Design review of the part built by this model. Coordinates are the model's own, in mm. Face numbers are marked on the shaded views. A direction names the side the tool comes from. Coordinates: 2 decimals unless noted, no trailing zeros. Loops run counter-clockwise (first coordinate to the right, second up) from the corner with the lowest first, then second, coordinate; pieces in that order, holes last. Notation, with made-up numbers: (-5, -15) -> (29, -15) arc R25 cw to (29, 7) -> close; hole circle Ø11 at (39.5, 38). An arc over 180 degrees is marked (long way). Answer as a JSON object with one key per item and string values.
```python
from build123d import *

# Parameters (mm, degrees)
BOSS_EXTRU_1_DEPTH      = 20
ESQUISSE2_R             = 1.25
ENL_V_MAT_EXTRU_1_DEPTH = 8
CONG_1_R                = 10
ESQUISSE3_R             = 2.5
ENL_V_MAT_EXTRU_2_DEPTH = 30


with BuildPart() as part:
    # Esquisse1 → Boss.-Extru.1 (new body)
    with BuildSketch(Plane.XY):
        with BuildLine():
            Line((-15, -0.5), (-15, -10))
            Line((-15, -10), (-12, -10))
            Line((-12, -10), (-12, -30))
            Line((-12, -30), (-9, -30))
            Line((-9, -30), (-9, -10))
            Line((-9, -10), (-6, -10))
            Line((-6, -10), (-6, -30))
            Line((-6, -30), (-3, -30))
            Line((-3, -30), (-3, -10))
            Line((-3, -10), (0, -10))
            Line((0, -10), (0, -30))
            Line((0, -30), (3, -30))
            Line((3, -30), (3, -10))
            Line((3, -10), (6, -10))
            Line((6, -10), (6, -30))
            Line((6, -30), (9, -30))
            Line((9, -30), (9, -10))
            Line((9, -10), (12, -10))
            Line((12, -10), (12, -30))
            Line((12, -30), (15, -30))
            Line((15, -30), (15, -0.5))
            Line((15, -0.5), (5.979130372, -0.5))
            ThreePointArc((5.979130372, -0.5), (0, -6), (-5.979130372, -0.5))
            Line((-5.979130372, -0.5), (-15, -0.5))
        make_face()
    extrude(amount=BOSS_EXTRU_1_DEPTH)

    # Esquisse2 → Enlèv. mat.-Extru.1 (cut)
    with BuildSketch(Plane(origin=(0, -0.5, 0), x_dir=(1, 0, 0), z_dir=(0, 1, 0))):
        with Locations(Location((-10, -5, 0), (0, 0, 180))):
            Circle(ESQUISSE2_R)
        with Locations(Location((-10, -15, 0), (0, 0, 180))):
            Circle(ESQUISSE2_R)
        with Locations(Location((10, -5, 0), (0, 0, 180))):
            Circle(ESQUISSE2_R)
        with Locations(Location((10, -15, 0), (0, 0, 180))):
            Circle(ESQUISSE2_R)
    extrude(amount=-ENL_V_MAT_EXTRU_1_DEPTH, mode=Mode.SUBTRACT)

    # Congé1
    cong_1_edges = [part.edges().sort_by_distance(p)[0] for p in [
        (-10.5, -30, 0),
        (-4.5, -30, 0),
        (1.5, -30, 0),
        (7.5, -30, 0),
        (13.5, -30, 0),
        (13.5, -30, 20),
        (7.5, -30, 20),
        (1.5, -30, 20),
        (-4.5, -30, 20),
        (-10.5, -30, 20),
    ]]
    fillet(cong_1_edges, radius=CONG_1_R - 0.0001)  # a hair under: the kernel refuses the full size

    # Esquisse3 → Enlèv. mat.-Extru.2 (cut)
    with BuildSketch(Plane(origin=(15, 0, 0), x_dir=(0, 0, -1), z_dir=(1, 0, 0))):
        with Locations(Location((-10, -20, 0), (0, 0, 90))):
            Circle(ESQUISSE3_R)
    extrude(amount=-ENL_V_MAT_EXTRU_2_DEPTH, mode=Mode.SUBTRACT)


solid = part.part
```
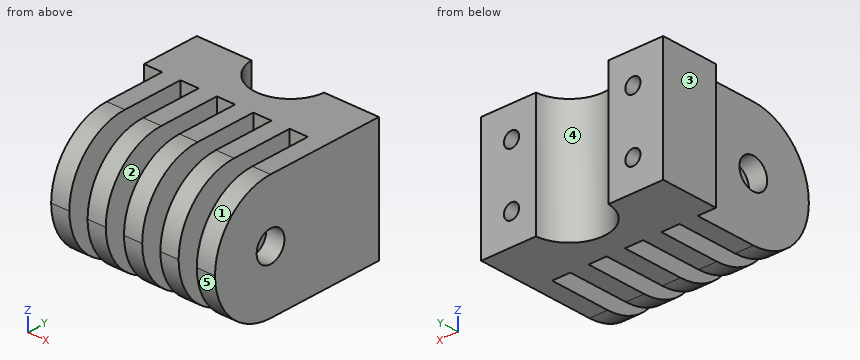
1) For the marked faces 1 and 2, list the 3-axis set-ups (+Z, -Z, +X, -X, +Y, -Y) from which the entire face can be reached by the end or side of a thin tool; tool diameter is ignored.
Completed:
{"face 1": "+Z, +X, -X, -Y", "face 2": "+Z, -Z, -Y"}
2) Add section D-D, the plane z = 18.25. Give the boundary of the cut face in (x, y), and give its area (3 significant figures).
Completed:
{"outline": "(-15, -10) -> (-12, -10) -> (-12, -25.65) -> (-9, -25.65) -> (-9, -10) -> (-6, -10) -> (-6, -25.65) -> (-3, -25.65) -> (-3, -10) -> (0, -10) -> (0, -25.65) -> (3, -25.65) -> (3, -10) -> (6, -10) -> (6, -25.65) -> (9, -25.65) -> (9, -10) -> (12, -10) -> (12, -25.65) -> (15, -25.65) -> (15, -0.5) -> (5.98, -0.5) arc R6 cw to (-5.98, -0.5) -> (-15, -0.5) -> close", "area": "469 mm²"}
3) Add section A-A, the plane y = -15.5. Give the boundary of the cut face in (x, z).
Completed:
{"outline": "(-12, 0) -> (-9, 0) -> (-9, 20) -> (-12, 20) -> close; (-6, 0) -> (-3, 0) -> (-3, 20) -> (-6, 20) -> close; (0, 0) -> (3, 0) -> (3, 20) -> (0, 20) -> close; (6, 0) -> (9, 0) -> (9, 20) -> (6, 20) -> close; (12, 0) -> (15, 0) -> (15, 20) -> (12, 20) -> close"}
4) Clearance check with flat-ended pins moving along their axes: pin 1 Ø1.5 at (y, z) = (-12.5, 10.5) entering from -X; pin 2 Ø4.5 at (y, z) = (-20, 10) entering from +X (3 decimals); pin 3 Ø3 at (x, z) = (-9.5, 15) entering from +Y; pin 4 Ø2 at (x, z) = (10, 15) entering from +Y. State where each tip first meets the part, or that it passes through.
Completed:
{"pin 1": "x = -12", "pin 2": "through", "pin 3": "y = -0.5", "pin 4": "y = -8.5"}
5) Add section C-C, the plane x = 10. Give the boundary of the cut face in (y, z), and give its area (3 significant figures).
Completed:
{"outline": "(-10, 0) -> (-0.5, 0) -> (-0.5, 3.75) -> (-8.5, 3.75) -> (-8.5, 6.25) -> (-0.5, 6.25) -> (-0.5, 13.75) -> (-8.5, 13.75) -> (-8.5, 16.25) -> (-0.5, 16.25) -> (-0.5, 20) -> (-10, 20) -> close", "area": "150 mm²"}
6) Wall thickness on probe 1 along Z at (x, y) = (10, -4.25); probe 2 along X at (y, z) = (-11, 9); probe 3 along Z at (x, y) = (14.15, -20): over which ranges is each line inside the solid? List them lowest first.
Completed:
{"probe 1": "0 to 3.75, 6.25 to 13.75, 16.25 to 20", "probe 2": "-12 to -9, -6 to -3, 0 to 3, 6 to 9, 12 to 15", "probe 3": "0 to 7.5, 12.5 to 20"}
7) The part is to be moulded in two halves that separate along X. For the marked faces 3, 4 and 5, say which applies: pulls with the +X half, pulls with the -X half, needs draft (parallel to the pull), parting line crosses it, or undercut.
Completed:
{"face 3": "pulls with the -X half", "face 4": "undercut", "face 5": "needs draft"}
